from build123d import *

# Parameters (mm, degrees)
BOSS_EXTRUDE1_DEPTH = 3
SKETCH3_W           = 27
SKETCH3_H           = 3.5
BOSS_EXTRUDE2_DEPTH = 16
SKETCH4_R           = 1.75
CUT_EXTRUDE1_DEPTH  = 10
SKETCH5_W           = 12
SKETCH5_H           = 8
CUT_EXTRUDE2_DEPTH  = 21


with BuildPart() as part:
    # Sketch2 → Boss-Extrude1 (new body)
    with BuildSketch(Plane.YZ):
        Polygon((-5, 66), (5, 66), (5, 16), (13.5, 16), (13.5, 0), (-13.5, 0), (-13.5, 16), (-5, 16), align=None)
        with BuildLine():
            Line((0.85, 53), (0.85, 17))
            ThreePointArc((0.85, 17), (-1, 15.15), (-2.85, 17))
            Line((-2.85, 17), (-2.85, 53))
            ThreePointArc((-2.85, 53), (-1, 54.85), (0.85, 53))
        make_face(mode=Mode.SUBTRACT)
    extrude(amount=BOSS_EXTRUDE1_DEPTH)

    # Sketch3 → Boss-Extrude2 (add)
    with BuildSketch(Plane.YZ.offset(3)):
        with Locations((0, 1.75)):
            Rectangle(SKETCH3_W, SKETCH3_H)
    extrude(amount=BOSS_EXTRUDE2_DEPTH)

    # Sketch4 → Cut-Extrude1 (cut)
    with BuildSketch(Plane.XY.offset(3.5)):
        with Locations((15, 9)):
            Circle(SKETCH4_R)
        with Locations((15, -9)):
            Circle(SKETCH4_R)
    extrude(amount=-CUT_EXTRUDE1_DEPTH, mode=Mode.SUBTRACT)

    # Sketch5 → Cut-Extrude2 (cut)
    with BuildSketch(Plane.YZ.offset(19)):
        with Locations((0, 4)):
            Rectangle(SKETCH5_W, SKETCH5_H)
    extrude(amount=-CUT_EXTRUDE2_DEPTH, mode=Mode.SUBTRACT)


solid = part.part
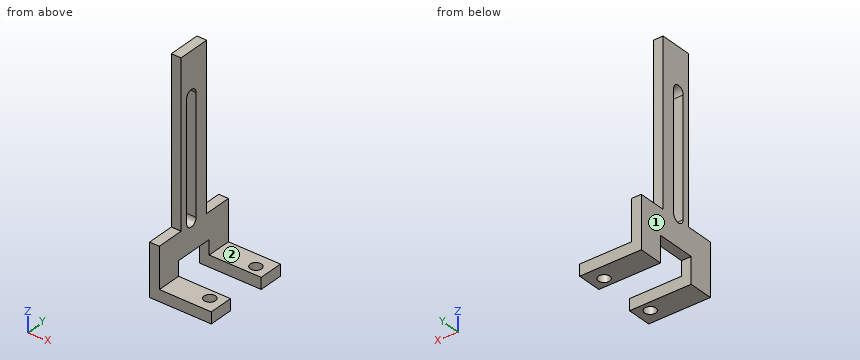
CAD build for the part. Positions are in the model's coordinates, mm. Face numbers are marked on the shaded views. A direction names the side the tool comes from. Round coordinates to 2 decimals unless told otherwise and drop trailing zeros. Order: outer loops, then holes, each group sorted by start corner. A loop starts at its lowest first (then second) coordinate and runs counter-clockwise, first axis right, second up. Notation, with made-up numbers: (57.5, 74.25) -> (73.5, 74.25) arc R20 ccw to (73.5, 90.25) -> close; hole circle Ø11 at (-34, -12.5). An arc over 180 degrees is marked (long way). Write item = value, one per line. Start each with the question number.
(1) Cut at D-D, the plane x = 15. List the corners of the cut face in (y, z).
(2) Pin check, flat tips, straight feed: P1, Ø1.5, axis at x = 3.5, y = 8, coming from the +Z side; P2, Ø3.5, axis at x = 1.5, y = -0.5, coming from the -Z side; P3, Ø1.5, axis at x = 1.5, z = 37.5, coming from the -Y side; P4, Ø4, axis at x = 5.5, z = 26, coming from the +Y side. Stop position of each tip, or through.
(3) Which spindle directions (+Z, -Z, +X, -X, +Y, -Y) get a long thin tool onto all of the face, cutting with end or side? Do the marked faces 1 and 2. Say none if no direction does.
(4) Probe line 1 (Y direction, x = 15, z = 2.35); line 2 (Y direction, x = 2.5, z = 34); line 3 (Z direction, x = 17.75, y = 11.25). List the from-to ranges inside material, lowest first. Write a range as [from, to].
(5) Cut at B-B, the plane y = 9. List the corners of the cut face in (x, z), then the cut area to 4 significant figures.
(6) Cut at A-A, the plane x = 10.25. List the corners of the cut face in (y, z), then the cut area to 3 significant figures.
(7) Cut at C-C, the plane z = 6.5. List the corners of the cut face in (x, y).
Model answer:
q1.outline = (-13.5, 0) -> (-10.75, 0) -> (-10.75, 3.5) -> (-13.5, 3.5) -> close; (-7.25, 0) -> (-6, 0) -> (-6, 3.5) -> (-7.25, 3.5) -> close; (6, 0) -> (7.25, 0) -> (7.25, 3.5) -> (6, 3.5) -> close; (10.75, 0) -> (13.5, 0) -> (13.5, 3.5) -> (10.75, 3.5) -> close
q2.P1 = 16
q2.P2 = 8
q2.P3 = -5
q2.P4 = through
q3.face_1 = +Z, -Z, -X, +Y, -Y
q3.face_2 = +Z, +X, +Y, -Y
q4.line_1 = [-13.5, -10.75], [-7.25, -6], [6, 7.25], [10.75, 13.5]
q4.line_2 = [-5, -2.85], [0.85, 5]
q4.line_3 = [0, 3.5]
q5.outline = (0, 0) -> (13.25, 0) -> (13.25, 3.5) -> (3, 3.5) -> (3, 16) -> (0, 16) -> close; (16.75, 0) -> (19, 0) -> (19, 3.5) -> (16.75, 3.5) -> close
q5.area = 91.75 mm2
q6.outline = (-13.5, 0) -> (-6, 0) -> (-6, 3.5) -> (-13.5, 3.5) -> close; (6, 0) -> (13.5, 0) -> (13.5, 3.5) -> (6, 3.5) -> close
q6.area = 52.5 mm2
q7.outline = (0, -13.5) -> (3, -13.5) -> (3, -6) -> (0, -6) -> close; (0, 6) -> (3, 6) -> (3, 13.5) -> (0, 13.5) -> close
